Here's how the part is built. I have some questions about the finished solid (model axes, mm). Face numbers are marked on the shaded views. A direction names the side the tool comes from. Coordinates: 2 decimals unless noted, no trailing zeros. Write each loop counter-clockwise with the first axis right and the second up, starting at its lowest first coordinate (ties: lowest second). Pieces come first, ordered by that corner, then holes. Notation, with made-up numbers: (-8.75, 38) -> (-0.75, 38) arc R16 cw to (-0.75, 57) -> close; hole circle Ø1 at (-14, -12.5). An arc over 180 degrees is marked (long way). Use a Markdown table: item, result. Add a question column.
Item 1: Imagine slicing it at C-C, the plane z = -33. Write out the boundary of the cut face in (x, y).
Item 2: If we mould it in two halves opening along X, with no side actions, what happens to the marked faces 3, 4, 5 and 6? For each: pulls with the +X half, pulls with the -X half, needs draft (parallel to the pull), parting line crosses it, or undercut.
Item 3: Will these pins go through, and if not, where does the flat tip stop? pin 1 Ø4 at (x, z) = (-4.5, -21.5) entering from +Y; pin 2 Ø0.9 at (x, z) = (0, -40) entering from +Y.
Item 4: If I drill on line 1 along Z through (x, y) = (0, -2.5); line 2 along X through (y, z) = (-60, 13); line 3 along Z through (x, y) = (-13, -133), over which ranges is the centre line in solid material (lowest first)? Write a range as from..to.
Item 5: Imagine slicing it at B-B, the plane x = -14.5. Write out the boundary of the cut face in (y, z).
Item 6: On a 3-axis mill with a long thin cutter (end or side, diameter ignored), from which of +Z, -Z, +X, -X, +Y, -Y can I reach the whole of each face in a straight line? I mean the marked faces 1 and 2. Say none if no direction works.
Item 7: Imagine slicing it at A-A, the plane y = -24. Write out the boundary of the cut face in (x, z).
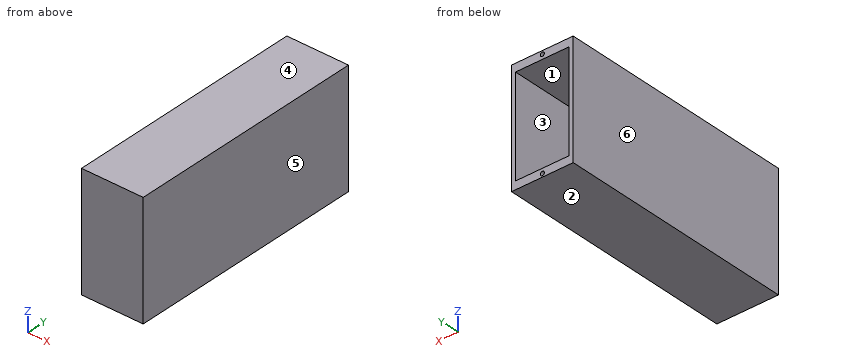
```python
from build123d import *

# Parameters (mm, degrees)
F0_W     = 46
F0_H     = 86
F1_DEPTH = 179
F2_W     = 40
F2_H     = 74
F3_DEPTH = 176
F4_R     = 1.5
F5_DEPTH = 8


with BuildPart() as f1:
    # F0 (on Front) → F1 (new body)
    with BuildSketch(Plane.XZ):
        Rectangle(F0_W, F0_H)
    extrude(amount=F1_DEPTH)

    # F2 (on face) → F3 (cut)
    with BuildSketch(Plane(origin=(0, 0, 0), x_dir=(-1, 0, 0), z_dir=(0, 1, 0))):
        Rectangle(F2_W, F2_H)
    extrude(amount=-F3_DEPTH, mode=Mode.SUBTRACT)

    # F4 (on face) → F5 (cut)
    with BuildSketch(Plane(origin=(0, 0, 0), x_dir=(-1, 0, 0), z_dir=(0, 1, 0))):
        with Locations((0, 40.5)):
            Circle(F4_R)
        with Locations((0, -40.5)):
            Circle(F4_R)
    extrude(amount=-F5_DEPTH, mode=Mode.SUBTRACT)


solid = f1.part
```
Ans:
| question | item | result |
|---|---|---|
| 1 | outline | (-23, -179) -> (23, -179) -> (23, 0) -> (20, 0) -> (20, -176) -> (-20, -176) -> (-20, 0) -> (-23, 0) -> close |
| 2 | face 3 | undercut |
| 2 | face 4 | needs draft |
| 2 | face 5 | pulls with the +X half |
| 2 | face 6 | pulls with the -X half |
| 3 | pin 1 | stops at y = -176 |
| 3 | pin 2 | stops at y = -8 |
| 4 | line 1 | z = -43..-42, -39..-37, 37..39, 42..43 |
| 4 | line 2 | x = -23..-20, 20..23 |
| 4 | line 3 | z = -43..-37, 37..43 |
| 5 | outline | (-179, -43) -> (0, -43) -> (0, -37) -> (-176, -37) -> (-176, 37) -> (0, 37) -> (0, 43) -> (-179, 43) -> close |
| 6 | face 1 | +Y |
| 6 | face 2 | -Z, +X, -X, +Y, -Y |
| 7 | outline | (-23, -43) -> (23, -43) -> (23, 43) -> (-23, 43) -> close; hole (-20, -37) -> (20, -37) -> (20, 37) -> (-20, 37) -> close |
